```python
from build123d import *

# Parameters (mm, degrees)
BOSS_EXTRUDE1_DEPTH = 20
SKETCH3_R           = 8
SKETCH3_R_2         = 1
CUT_EXTRUDE1_DEPTH  = 10
SKETCH4_R           = 1
CUT_EXTRUDE2_DEPTH  = 10
SKETCH5_R           = 2
CUT_EXTRUDE3_DEPTH  = 2
SKETCH6_W           = 17
SKETCH6_H           = 1
CUT_EXTRUDE4_DEPTH  = 65


with BuildPart() as part:
    # Sketch1 → Boss-Extrude1 (new body)
    with BuildSketch(Plane(origin=(0, 0, 0), x_dir=(0, 0, -1), z_dir=(1, 0, 0))):
        Polygon((0, 0), (20.5, 0), (20.5, 40), (25.5, 40), (25.5, -5), (0, -5), align=None)
    extrude(amount=BOSS_EXTRUDE1_DEPTH)

    # Sketch3 → Cut-Extrude1 (cut)
    with BuildSketch(Plane(origin=(0, 0, 0), x_dir=(1, 0, 0), z_dir=(0, 1, 0))):
        with Locations(Location((10, 10, 0), (0, 0, 270))):
            Circle(SKETCH3_R)
        with Locations(Location((2.3, 17.7, 0), (0, 0, 270))):
            Circle(SKETCH3_R_2)
        with Locations(Location((17.7, 17.7, 0), (0, 0, 270))):
            Circle(SKETCH3_R_2)
        with Locations(Location((17.7, 2.3, 0), (0, 0, 270))):
            Circle(SKETCH3_R_2)
        with Locations(Location((2.3, 2.3, 0), (0, 0, 270))):
            Circle(SKETCH3_R_2)
    extrude(amount=-CUT_EXTRUDE1_DEPTH, mode=Mode.SUBTRACT)

    # Sketch4 → Cut-Extrude2 (cut)
    with BuildSketch(Plane.XY.offset(-20.5)):
        with Locations((5.5, 15)):
            Circle(SKETCH4_R)
        with Locations((5.5, 23)):
            Circle(SKETCH4_R)
        with Locations((17.5, 23)):
            Circle(SKETCH4_R)
        with Locations((17.5, 15)):
            Circle(SKETCH4_R)
    extrude(amount=-CUT_EXTRUDE2_DEPTH, mode=Mode.SUBTRACT)

    # Sketch5 → Cut-Extrude3 (cut)
    with BuildSketch(Plane.XY.offset(-20.5)):
        with Locations((5.5, 23)):
            Circle(SKETCH5_R)
        with Locations((5.5, 15)):
            Circle(SKETCH5_R)
        with Locations((17.5, 15)):
            Circle(SKETCH5_R)
        with Locations((17.5, 23)):
            Circle(SKETCH5_R)
    extrude(amount=-CUT_EXTRUDE3_DEPTH, mode=Mode.SUBTRACT)

    # Sketch6 → Cut-Extrude4 (cut)
    with BuildSketch(Plane(origin=(0, 40, 0), x_dir=(1, 0, 0), z_dir=(0, 1, 0))):
        with Locations((11.5, 25)):
            Rectangle(SKETCH6_W, SKETCH6_H)
    extrude(amount=-CUT_EXTRUDE4_DEPTH, mode=Mode.SUBTRACT)


solid = part.part
```
CAD build for the part. Positions are in the model's coordinates, mm. A direction names the side the tool comes from. Round coordinates to 2 decimals unless told otherwise and drop trailing zeros. Write each loop counter-clockwise with the first axis right and the second up, starting at its lowest first coordinate (ties: lowest second). Pieces come first, ordered by that corner, then holes. Notation, with made-up numbers: M -36.5,60 L -17.5,60 A27 cw -17.5,83 Z; hole C -25,39 d11. An arc over 180 degrees is marked long. One line per question, with ' | ' between items.
1. Cut at C-C on z = -4. Write the cut outline in (x, y).
Working result:
outline: M 0,-5 L 4.71,-5 L 4.71,0 L 0,0 Z; M 15.29,-5 L 20,-5 L 20,0 L 15.29,0 Z
2. Cut at D-D on x = 5.5. Write the cut outline in (y, z).
Working result:
outline: M -5,-24.5 L 14,-24.5 L 14,-22.5 L 13,-22.5 L 13,-20.5 L 0,-20.5 L 0,-16.61 L -5,-16.61 Z; M -5,-3.39 L 0,-3.39 L 0,0 L -5,0 Z; M 16,-24.5 L 22,-24.5 L 22,-22.5 L 21,-22.5 L 21,-20.5 L 17,-20.5 L 17,-22.5 L 16,-22.5 Z; M 24,-24.5 L 40,-24.5 L 40,-20.5 L 25,-20.5 L 25,-22.5 L 24,-22.5 Z
3. Cut at B-B on x = 10. Write the cut outline in (y, z).
Working result:
outline: M -5,-24.5 L 40,-24.5 L 40,-20.5 L 0,-20.5 L 0,-18 L -5,-18 Z; M -5,-2 L 0,-2 L 0,0 L -5,0 Z
4. Mould opens along Z. For faces 4 (the cylindrical face through (17.96, 14.11, -23.49)), 5 (the cylindrical face through (16.724, -2.465, -2.517)), 6 (the flat face through (10, 20, -20.5)) say: pulls with the +Z half, pulls with the -Z half, needs draft (parallel to the pull), parting line crosses it, or undercut.
Working result:
face 4: needs draft | face 5: undercut | face 6: pulls with the +Z half
5. Probe L1, parallel to Y at x = 5.5, z = -23.1; L2, parallel to Z at x = 12, y = 5; L3, parallel to Y at x = 3.5, z = -3. List the from-to ranges inside material, lowest first. Write a range as from..to.
Working result:
L1: -5..14, 16..22, 24..40 | L2: -24.5..-20.5 | L3: -5..0
6. Pin check, flat tips, straight feed: pin 1 Ø2.5 at (x, z) = (2.3, -2.3) entering from +Y; pin 2 Ø2.5 at (x, y) = (17.5, 23) entering from -Z; pin 3 Ø4.5 at (x, y) = (4.5, 23) entering from +Z. Stop position of each tip, or through.
Working result:
pin 1: y = 0 | pin 2: z = -24.5 | pin 3: z = -20.5
7. Which spindle directions (+Z, -Z, +X, -X, +Y, -Y) get a long thin tool onto all of the face, cutting with end or side? Do faces 1 (the flat face through (3, 18, -25)), 2 (the flat face through (3, 0, -15)), 3 (the cylindrical face through (17.24, 16.983, -21.486)). Say none if no direction does.
Working result:
face 1: -Z, +X, +Y, -Y | face 2: +Z, +X, -X, +Y | face 3: +Z
8. Cut at A-A on y = 15. Write the cut outline in (x, z), and give its area (3 significant figures).
Working result:
outline: M 0,-25.5 L 3,-25.5 L 3,-24.5 L 4.5,-24.5 L 4.5,-22.5 L 3.5,-22.5 L 3.5,-20.5 L 0,-20.5 Z; M 6.5,-24.5 L 16.5,-24.5 L 16.5,-22.5 L 15.5,-22.5 L 15.5,-20.5 L 7.5,-20.5 L 7.5,-22.5 L 6.5,-22.5 Z; M 18.5,-24.5 L 20,-24.5 L 20,-20.5 L 19.5,-20.5 L 19.5,-22.5 L 18.5,-22.5 Z | area: 59.0 mm2
